Autodesk Inventor part; units mm, degrees
ref_plane "YZ Plane" through (0, 0, 0) normal (1, 0, 0) x (0, 1, 0)
ref_plane "XZ Plane" through (0, 0, 0) normal (0, 1, 0) x (-1, 0, 0)
ref_plane "XY Plane" through (0, 0, 0) normal (0, 0, 1) x (1, 0, 0)
sketch "Sketch1" plane through (0, 0, 0) normal (0, 0, 1) x (1, 0, 0)
  circle A0 centre (1.016, 0) radius 19.05
  line L0 (159.5437, -28.575) -> (159.5437, 29.0493)
  line L1 (145.8277, 86.9876) -> (-55.3403, 86.9876)
  line L2 (159.5437, 93.3376) -> (-107.1563, 93.3376)
  line L3 (-107.1563, 93.3376) -> (-107.1563, -59.0624)
  line L4 (-107.1563, -59.0624) -> (159.5437, -59.0624)
  line L5 (159.5437, -59.0624) -> (159.5437, 93.3376)
  point P0 (0, 0)
  dimension "d0" = 266.7
  dimension "d1" = 152.4
  dimension "d15" = 38.1
extrude "Extrusion1" add sketch "Sketch1" along normal blind 6.35
sketch "Sketch2" plane through (0, 0, 6.35) normal (0, 0, 1) x (1, 0, 0)
  line L0 (-107.1563, 93.3376) -> (159.5437, 93.3376)
  line L1 (-107.1563, -59.0624) -> (-107.1563, 93.3376)
  line L2 (-103.9813, 93.3376) -> (-103.9813, -59.0624) construction
  circle A0 centre (-103.9813, 80.6376) radius 1.8542
  dimension "d4" = 3.175
  dimension "d5" = 3.7084
  dimension "d6" = 12.7
extrude "Extrusion2" cut sketch "Sketch2" against normal through all
pattern_linear "Rectangular Pattern1" count 2 spacing 127 along (0, -1, 0) count 2 spacing 260.35 along (1, 0, 0) of "Extrusion2"
sketch "Sketch3" plane through (0, 0, 0) normal (0, 0, -1) x (-1, 0, 0)
  circle A0 centre (62.484, 38.1) radius 2.5146
  circle A1 centre (62.484, -38.1) radius 2.5146
  circle A2 centre (-115.316, -38.1) radius 2.5146
  circle A3 centre (-115.316, 38.1) radius 2.5146
  point P0 (0, 0)
extrude "Extrusion3" cut sketch "Sketch3" against normal through all
sketch "Sketch4" plane through (0, 0, 0) normal (0, 0, -1) x (-1, 0, 0)
  line L0 (107.1563, 93.3376) -> (113.5063, 93.3376)
  line L1 (113.5063, 93.3376) -> (113.5063, -59.0624)
  line L2 (113.5063, -59.0624) -> (107.1563, -59.0624)
  line L3 (107.1563, -59.0624) -> (107.1563, 93.3376)
  line L4 (-159.5437, -59.0624) -> (-165.8937, -59.0624)
  line L5 (-165.8937, -59.0624) -> (-165.8937, 93.3376)
  line L6 (-165.8937, 93.3376) -> (-159.5437, 93.3376)
  line L7 (-159.5437, 93.3376) -> (-159.5437, -59.0624)
  point P0 (0, 0)
  dimension "d18" = 6.35
  dimension "d19" = 6.35
extrude "Extrusion4" add sketch "Sketch4" against normal blind 6.35
sketch "Sketch5" plane through (0, 0, 0) normal (0, 0, -1) x (-1, 0, 0)
  line L0 (-159.5437, -59.0624) -> (-159.5437, 93.3376)
  line L1 (-159.5437, 93.3376) -> (-153.1937, 93.3376)
  line L2 (-153.1937, -59.0624) -> (-153.1937, 93.3376)
  line L3 (-159.5437, -59.0624) -> (-153.1937, -59.0624)
  line L4 (-159.5437, 68.2942) -> (-153.1937, 68.2942)
  line L5 (-153.1937, 68.2942) -> (-153.1937, 42.8942)
  line L6 (-153.1937, 42.8942) -> (-159.5437, 42.8942)
  line L7 (-159.5437, 42.8942) -> (-159.5437, 68.2942)
  line L8 (-159.5437, -7.9058) -> (-153.1937, -7.9058)
  line L9 (-153.1937, -7.9058) -> (-153.1937, -33.3058)
  line L10 (-153.1937, -33.3058) -> (-159.5437, -33.3058)
  line L11 (-159.5437, -33.3058) -> (-159.5437, -7.9058)
  line L12 (100.8063, 68.2942) -> (107.1563, 68.2942)
  line L13 (107.1563, 68.2942) -> (107.1563, 42.8942)
  line L14 (107.1563, 42.8942) -> (100.8063, 42.8942)
  line L15 (100.8063, 42.8942) -> (100.8063, 68.2942)
  line L16 (100.8063, -7.9058) -> (107.1563, -7.9058)
  line L17 (107.1563, -7.9058) -> (107.1563, -33.3058)
  line L18 (107.1563, -33.3058) -> (100.8063, -33.3058)
  line L19 (100.8063, -33.3058) -> (100.8063, -7.9058)
  point P0 (0, 0)
  dimension "d22" = 25.4
  dimension "d25" = 76.2
  dimension "d28" = 260.35
extrude "Extrusion5" cut sketch "Sketch5" against normal through all contours L0 L8 L2 L10 | L0 L4 L2 L6 | L12 L13 L14 L15 | L16 L17 L18 L19
properties part number "panStepperMountRB01" material "Wood (Oak)"
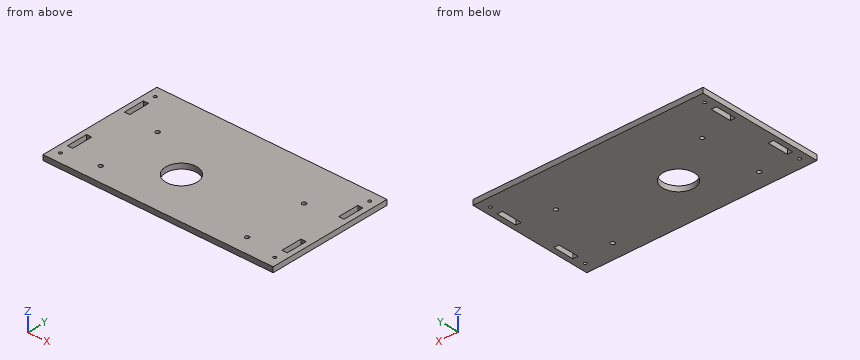
Can you work these out from the model? Positions are in its coordinate system, mm. Round coordinates to 2 decimals unless told otherwise and drop trailing zeros. Order: outer loops, then holes, each group sorted by start corner. A loop starts at its lowest first (then second) coordinate and runs counter-clockwise, first axis right, second up. Notation, with made-up numbers: (55.25, 0) -> (94.25, 0) arc R13 cw to (94.25, 23) -> close; hole circle Ø2 at (-21.5, -34.75). An arc over 180 degrees is marked (long way). Return JSON: item names as keys, results as strings. Group by question number.
1. If we section it at C-C, the plane z = 1.5: Count the separate pieces of the cut face and the enclosed holes in it, then the cut area to 3 significant figures.
2. If we section it at A-A, the plane y = 0: Write out the boundary of the cut face in (x, z), then the cut area to 3 significant figures.
3. If we section it at B-B, the plane x = -14: Write out the boundary of the cut face in (y, z).
4. I need wall thicknesses on line 1 (X direction, y = -33, z = 5.5); line 2 (X direction, y = -38.5, z = 2.5); line 3 (Y direction, x = 115, z = 4.5). Which ranges of each line are inside material? Lowest first, please. Write a range as [from, to].
Output values:
{
 "1": {"separate pieces": "1", "enclosed holes": "13", "area": "40,700 mm²"},
 "2": {"outline": "(-113.51, 0) -> (-18.03, 0) -> (-18.03, 6.35) -> (-113.51, 6.35) -> close; (20.07, 0) -> (165.89, 0) -> (165.89, 6.35) -> (20.07, 6.35) -> close", "area": "1,530 mm²"},
 "3": {"outline": "(-59.06, 0) -> (-11.72, 0) -> (-11.72, 6.35) -> (-59.06, 6.35) -> close; (11.72, 0) -> (93.34, 0) -> (93.34, 6.35) -> (11.72, 6.35) -> close"},
 "4": {"line 1": "[-113.51, -107.16], [-100.81, 153.19], [159.54, 165.89]", "line 2": "[-113.51, -64.97], [-60, 112.83], [117.8, 165.89]", "line 3": "[-59.06, -40.59], [-35.61, 35.61], [40.59, 93.34]"}
}
